Build history of the part. All positions in model axes, mm. Face numbers are marked on the shaded views. A direction names the side the tool comes from. Coordinates: 2 decimals unless noted, no trailing zeros. Loops run counter-clockwise (first coordinate to the right, second up) from the corner with the lowest first, then second, coordinate; pieces in that order, holes last. Notation, with made-up numbers: (-13.75, 15.25) -> (41.25, 15.25) arc R19 ccw to (41.25, 28.25) -> close; hole circle Ø1 at (1.25, -19.75). An arc over 180 degrees is marked (long way). One line per item, written item: value. Start each with the question number.
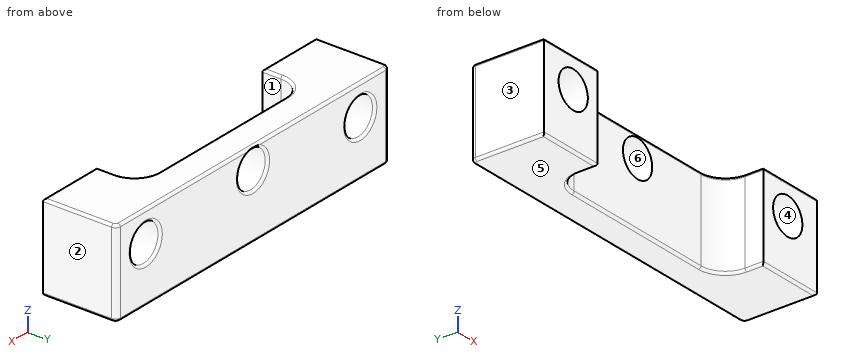
```python
from build123d import *

# Parameters (mm, degrees)
BOSS_EXTRUDE1_DEPTH = 3.5
SKETCH2_R           = 1.5
CUT_EXTRUDE1_DEPTH  = 16.628499608
FILLET1_R           = 2
FILLET2_R           = 0.4
FILLET3_R           = 0.2


with BuildPart() as part:
    # Sketch1 → Boss-Extrude1 (new, symmetric)
    with BuildSketch(Plane.XY):
        Polygon((-14, 0), (-14, 6), (14, 6), (14, 0), (8.5, 0), (8.5, 3.5), (-8.5, 3.5), (-8.5, 0), align=None)
    extrude(amount=BOSS_EXTRUDE1_DEPTH, both=True)

    # Sketch2 → Cut-Extrude1 (cut, through all)
    with BuildSketch(Plane(origin=(0, 6, 0), x_dir=(1, 0, 0), z_dir=(0, 1, 0))):
        with Locations(Location((11, -1, 0), (0, 0, 270))):
            Circle(SKETCH2_R)
        with Locations(Location((-11, -1, 0), (0, 0, 90))):
            Circle(SKETCH2_R)
        with Locations(Location((0, -1.75, 0), (0, 0, 270))):
            Circle(SKETCH2_R)
    extrude(amount=-CUT_EXTRUDE1_DEPTH, mode=Mode.SUBTRACT)

    # Fillet1
    fillet1_edges = [part.edges().sort_by_distance(p)[0] for p in [
        (8.5, 3.5, 0),
        (-8.5, 3.5, 0),
    ]]
    fillet(fillet1_edges, radius=FILLET1_R)

    # Fillet2
    fillet2_edges = [part.edges().sort_by_distance(p)[0] for p in [
        (-14, 6, 0),
        (14, 6, 0),
    ]]
    fillet(fillet2_edges, radius=FILLET2_R)

    # Fillet3
    # the kernel refuses this fillet: 0.2 mm, written as the material it takes off along each edge
    with BuildSketch(Plane(origin=(-8.5, 1.5, -3.5), x_dir=(-1, 0, 0), z_dir=(0, -1, 0)), Plane(origin=(8.5, -0.5, -3.5), x_dir=(1, 0, 0), z_dir=(0, 1, 0)), Plane(origin=(8.5, -0.5, 3.5), x_dir=(0, 0, -1), z_dir=(0, 1, 0)), Plane(origin=(-8.5, 1.5, 3.5), x_dir=(0, 0, -1), z_dir=(0, -1, 0))) as fillet3_piece_1:
        with BuildLine():
            CenterArc((FILLET3_R, -FILLET3_R), FILLET3_R, 90, 90)
            Line((0, -FILLET3_R), (0, 0))
            Line((0, 0), (FILLET3_R, 0))
        make_face()
    extrude(amount=2, mode=Mode.SUBTRACT)
    with BuildSketch(Plane(origin=(-8, 0, -3.5), x_dir=(0, 1, 0), z_dir=(-1, 0, 0)), Plane(origin=(14.5, 0, 3.5), x_dir=(0, 0, -1), z_dir=(-1, 0, 0)), Plane(origin=(-8, 0, 3.5), x_dir=(0, 0, -1), z_dir=(-1, 0, 0)), Plane(origin=(14.5, 0, -3.5), x_dir=(0, 1, 0), z_dir=(-1, 0, 0))) as fillet3_piece_2:
        with BuildLine():
            CenterArc((FILLET3_R, -FILLET3_R), FILLET3_R, 90, 90)
            Line((0, -FILLET3_R), (0, 0))
            Line((0, 0), (FILLET3_R, 0))
        make_face()
    extrude(amount=6.5, mode=Mode.SUBTRACT)
    with BuildSketch(Plane(origin=(14, 5.6, 3.5), x_dir=(0, 0, -1), z_dir=(0, -1, 0)), Plane(origin=(-14, -0.5, -3.5), x_dir=(1, 0, 0), z_dir=(0, 1, 0)), Plane(origin=(-14, -0.5, 3.5), x_dir=(0, 0, -1), z_dir=(0, 1, 0)), Plane(origin=(14, 5.6, -3.5), x_dir=(-1, 0, 0), z_dir=(0, -1, 0))) as fillet3_piece_3:
        with BuildLine():
            CenterArc((FILLET3_R, -FILLET3_R), FILLET3_R, 90, 90)
            Line((0, -FILLET3_R), (0, 0))
            Line((0, 0), (FILLET3_R, 0))
        make_face()
    extrude(amount=6.1, mode=Mode.SUBTRACT)
    with BuildSketch(Plane(origin=(11, 6, 1), x_dir=(0, 0, 1), z_dir=(-1, 0, 0))) as fillet3_piece_4:
        with BuildLine():
            CenterArc((1.5 + FILLET3_R, -FILLET3_R), FILLET3_R, 90, 90)
            Line((1.5, -FILLET3_R), (1.5, 0))
            Line((1.5, 0), (1.5 + FILLET3_R, 0))
        make_face()
    revolve(axis=Axis((11, 6, 1), (0, 1, 0)), mode=Mode.SUBTRACT)
    with BuildSketch(Plane(origin=(-11, 6, 1), x_dir=(0, 0, -1), z_dir=(1, 0, 0))) as fillet3_piece_5:
        with BuildLine():
            CenterArc((1.5 + FILLET3_R, -FILLET3_R), FILLET3_R, 90, 90)
            Line((1.5, -FILLET3_R), (1.5, 0))
            Line((1.5, 0), (1.5 + FILLET3_R, 0))
        make_face()
    revolve(axis=Axis((-11, 6, 1), (0, 1, 0)), mode=Mode.SUBTRACT)
    with BuildSketch(Plane(origin=(0, 6, 1.75), x_dir=(0, 0, 1), z_dir=(-1, 0, 0))) as fillet3_piece_6:
        with BuildLine():
            CenterArc((1.5 + FILLET3_R, -FILLET3_R), FILLET3_R, 90, 90)
            Line((1.5, -FILLET3_R), (1.5, 0))
            Line((1.5, 0), (1.5 + FILLET3_R, 0))
        make_face()
    revolve(axis=Axis((0, 6, 1.75), (0, 1, 0)), mode=Mode.SUBTRACT)
    with BuildSketch(Plane(origin=(6.5, 3.5, -3.5), x_dir=(0, 1, 0), z_dir=(-1, 0, 0)), Plane(origin=(6.5, 3.5, 3.5), x_dir=(0, 0, -1), z_dir=(-1, 0, 0))) as fillet3_piece_7:
        with BuildLine():
            CenterArc((FILLET3_R, -FILLET3_R), FILLET3_R, 90, 90)
            Line((0, -FILLET3_R), (0, 0))
            Line((0, 0), (FILLET3_R, 0))
        make_face()
    extrude(amount=13, mode=Mode.SUBTRACT)
    with BuildSketch(Plane(origin=(6.5, 1.5, -3.5), x_dir=(1, 0, 0), z_dir=(0, -1, 0))) as fillet3_piece_8:
        with BuildLine():
            CenterArc((2 + FILLET3_R, FILLET3_R), FILLET3_R, 180, 90)
            Line((2, FILLET3_R), (2, 0))
            Line((2, 0), (2 + FILLET3_R, 0))
        make_face()
    revolve(axis=Axis((6.5, 1.5, -3.5), (0, 0, 1)), revolution_arc=90, mode=Mode.SUBTRACT)
    with BuildSketch(Plane(origin=(6.5, 1.5, 3.5), x_dir=(1, 0, 0), z_dir=(0, -1, 0))) as fillet3_piece_9:
        with BuildLine():
            CenterArc((2 + FILLET3_R, -FILLET3_R), FILLET3_R, 90, 90)
            Line((2 + FILLET3_R, 0), (2, 0))
            Line((2, 0), (2, -FILLET3_R))
        make_face()
    revolve(axis=Axis((6.5, 1.5, 3.5), (0, 0, 1)), revolution_arc=90, mode=Mode.SUBTRACT)
    with BuildSketch(Plane(origin=(-6.5, 1.5, -3.5), x_dir=(-1, 0, 0), z_dir=(0, -1, 0))) as fillet3_piece_10:
        with BuildLine():
            CenterArc((2 + FILLET3_R, -FILLET3_R), FILLET3_R, 90, 90)
            Line((2, -FILLET3_R), (2, 0))
            Line((2, 0), (2 + FILLET3_R, 0))
        make_face()
    revolve(axis=Axis((-6.5, 1.5, -3.5), (0, 0, -1)), revolution_arc=90, mode=Mode.SUBTRACT)
    with BuildSketch(Plane(origin=(-6.5, 1.5, 3.5), x_dir=(-1, 0, 0), z_dir=(0, -1, 0))) as fillet3_piece_11:
        with BuildLine():
            CenterArc((2 + FILLET3_R, FILLET3_R), FILLET3_R, 180, 90)
            Line((2 + FILLET3_R, 0), (2, 0))
            Line((2, 0), (2, FILLET3_R))
        make_face()
    revolve(axis=Axis((-6.5, 1.5, 3.5), (0, 0, -1)), revolution_arc=90, mode=Mode.SUBTRACT)
    with BuildSketch(Plane(origin=(-13.6, 6, -3.5), x_dir=(0, -1, 0), z_dir=(1, 0, 0)), Plane(origin=(-13.6, 6, 3.5), x_dir=(0, 0, -1), z_dir=(1, 0, 0))) as fillet3_piece_12:
        with BuildLine():
            CenterArc((FILLET3_R, -FILLET3_R), FILLET3_R, 90, 90)
            Line((0, -FILLET3_R), (0, 0))
            Line((0, 0), (FILLET3_R, 0))
        make_face()
    extrude(amount=27.2, mode=Mode.SUBTRACT)
    with BuildSketch(Plane(origin=(-13.6, 5.6, -3.5), x_dir=(0, 1, 0), z_dir=(1, 0, 0))) as fillet3_piece_13:
        with BuildLine():
            CenterArc((0.4 - FILLET3_R, FILLET3_R), FILLET3_R, 270, 90)
            Line((0.4, FILLET3_R), (0.4, 0))
            Line((0.4, 0), (0.4 - FILLET3_R, 0))
        make_face()
    revolve(axis=Axis((-13.6, 5.6, -3.5), (0, 0, 1)), revolution_arc=90, mode=Mode.SUBTRACT)
    with BuildSketch(Plane(origin=(13.6, 5.6, -3.5), x_dir=(1, 0, 0), z_dir=(0, -1, 0))) as fillet3_piece_14:
        with BuildLine():
            CenterArc((0.4 - FILLET3_R, FILLET3_R), FILLET3_R, 270, 90)
            Line((0.4, FILLET3_R), (0.4, 0))
            Line((0.4, 0), (0.4 - FILLET3_R, 0))
        make_face()
    revolve(axis=Axis((13.6, 5.6, -3.5), (0, 0, 1)), revolution_arc=90, mode=Mode.SUBTRACT)
    with BuildSketch(Plane(origin=(-13.6, 5.6, 3.5), x_dir=(0, 1, 0), z_dir=(1, 0, 0))) as fillet3_piece_15:
        with BuildLine():
            CenterArc((0.4 - FILLET3_R, -FILLET3_R), FILLET3_R, 0, 90)
            Line((0.4 - FILLET3_R, 0), (0.4, 0))
            Line((0.4, 0), (0.4, -FILLET3_R))
        make_face()
    revolve(axis=Axis((-13.6, 5.6, 3.5), (0, 0, 1)), revolution_arc=90, mode=Mode.SUBTRACT)
    with BuildSketch(Plane(origin=(13.6, 5.6, 3.5), x_dir=(1, 0, 0), z_dir=(0, -1, 0))) as fillet3_piece_16:
        with BuildLine():
            CenterArc((0.4 - FILLET3_R, -FILLET3_R), FILLET3_R, 0, 90)
            Line((0.4 - FILLET3_R, 0), (0.4, 0))
            Line((0.4, 0), (0.4, -FILLET3_R))
        make_face()
    revolve(axis=Axis((13.6, 5.6, 3.5), (0, 0, 1)), revolution_arc=90, mode=Mode.SUBTRACT)


solid = part.part
```
Item 1: Band-saw the part on D-D, the plane z = 1.75. Count the separate pieces of the cut face and the enclosed holes in it, and give its area (3 significant figures).
Item 2: Drop a flat-ended pin along its axis: pin 1 Ø3.5 at (x, z) = (-1.5, -0.5) entering from -Y. Give the stop position or say it passes through.
Item 3: Band-saw the part on C-C, the plane y = 4.75. List the corners of the cut face in (x, z), and give its area (3 significant figures).
Item 4: Band-saw the part on A-A, the plane y = 1. List the corners of the cut face in (x, z), and give its area (3 significant figures).
Item 5: Probe probe 1 along Z at (x, y) = (-11, 3.25); probe 2 along X at (y, z) = (3.9, 1); probe 3 along X at (y, z) = (1.9, 1). List the from-to ranges inside material, lowest first.
Item 6: Tool access for the marked faces 1 and 2: list every direction of +Z, -Z, +X, -X, +Y, -Y with a clear straight run to the whole face (end or side of a thin tool).
Item 7: Two-plate mould, pull along Z, no slides. Class the marked faces 3, 4, 5 and 6: +Z half, -Z half, draft (parallel to the pull), parting line (faces both ways), or undercut.
Item 8: Band-saw the part on B-B, the plane x = 11. List the corners of the cut face in (y, z).
Worked out:
1. separate pieces: 4
1. enclosed holes: 0
1. area: 71.4 mm²
2. pin 1: stops at y = 3.5
3. outline: (-14, -3.3) arc R0.2 ccw to (-13.8, -3.5) -> (13.8, -3.5) arc R0.2 ccw to (14, -3.3) -> (14, 3.3) arc R0.2 ccw to (13.8, 3.5) -> (-13.8, 3.5) arc R0.2 ccw to (-14, 3.3) -> close; hole circle Ø3 at (-11, 1); hole circle Ø3 at (0, 1.75); hole circle Ø3 at (11, 1)
3. area: 175 mm²
4. outline: (-14, -3.3) arc R0.2 ccw to (-13.8, -3.5) -> (-8.7, -3.5) arc R0.2 ccw to (-8.5, -3.3) -> (-8.5, 3.3) arc R0.2 ccw to (-8.7, 3.5) -> (-13.8, 3.5) arc R0.2 ccw to (-14, 3.3) -> close; (8.5, -3.3) arc R0.2 ccw to (8.7, -3.5) -> (13.8, -3.5) arc R0.2 ccw to (14, -3.3) -> (14, 3.3) arc R0.2 ccw to (13.8, 3.5) -> (8.7, 3.5) arc R0.2 ccw to (8.5, 3.3) -> close; hole circle Ø3 at (-11, 1); hole circle Ø3 at (11, 1)
4. area: 62.8 mm²
5. probe 1: z = -3.5 to -0.5, 2.5 to 3.5
5. probe 2: x = -14 to -12.5, -9.5 to -1.3, 1.3 to 9.5, 12.5 to 14
5. probe 3: x = -14 to -12.5, -9.5 to -8.46, 8.46 to 9.5, 12.5 to 14
6. face 1: +Z, -Z, -Y
6. face 2: +Z, -Z, +X, +Y, -Y
7. face 3: draft
7. face 4: undercut
7. face 5: -Z half
7. face 6: undercut
8. outline: (0, -3.3) arc R0.2 ccw to (0.2, -3.5) -> (5.8, -3.5) arc R0.2 ccw to (6, -3.3) -> (6, -0.7) arc R0.2 ccw to (5.8, -0.5) -> (0, -0.5) -> close; (0, 2.5) -> (5.8, 2.5) arc R0.2 ccw to (6, 2.7) -> (6, 3.3) arc R0.2 ccw to (5.8, 3.5) -> (0.2, 3.5) arc R0.2 ccw to (0, 3.3) -> close
